Source: CAD feature listing. Evaluate the final solid. Frame: model axes, mm. A direction names the side the tool comes from. Give positions to 0.01 mm unless a question says otherwise; leave off trailing zeros. Write each loop counter-clockwise with the first axis right and the second up, starting at its lowest first coordinate (ties: lowest second). Pieces come first, ordered by that corner, then holes. Notation, with made-up numbers: (4.5, 30.5) -> (14.5, 30.5) arc R34 ccw to (14.5, 60.5) -> close; hole circle Ø2 at (19, 1.5). An arc over 180 degrees is marked (long way). Write item = value, one per line.
from build123d import *

# Parameters (mm, degrees)
BOSS_EXTRUDE1_DEPTH     = 7.3
CUT_EXTRUDE1_DEPTH      = 8
CUT_EXTRUDE2_DEPTH      = 8
CUT_EXTRUDE3_DEPTH      = 34.01953967
CUT_EXTRUDE3_DEPTH_BACK = 34.01953967
CHAMFER1_SIZE           = 0.7


with BuildPart() as part:
    # Sketch1 → Boss-Extrude1 (new body)
    with BuildSketch(Plane.XY):
        Polygon((0, 0), (19, 0), (19, 18), (10.45, 18), (10.45, 26), (8.55, 26), (8.55, 18), (0, 18), align=None)
    extrude(amount=BOSS_EXTRUDE1_DEPTH)

    # Sketch2 → Cut-Extrude1 (cut)
    with BuildSketch(Plane(origin=(0, 26, 0), x_dir=(1, 0, 0), z_dir=(0, 1, 0))):
        with BuildLine():
            Line((8.55, -0.95), (8.55, 0))
            Line((8.55, 0), (9.5, 0))
            ThreePointArc((9.5, 0), (8.828248558, -0.278248558), (8.55, -0.95))
        make_face()
    extrude(amount=-CUT_EXTRUDE1_DEPTH, mode=Mode.SUBTRACT)

    # Sketch3 → Cut-Extrude2 (cut)
    with BuildSketch(Plane(origin=(0, 26, 0), x_dir=(1, 0, 0), z_dir=(0, 1, 0))):
        with BuildLine():
            Line((9.5, 0), (10.45, 0))
            Line((10.45, 0), (10.45, -0.95))
            ThreePointArc((10.45, -0.95), (10.171751442, -0.278248558), (9.5, 0))
        make_face()
    extrude(amount=-CUT_EXTRUDE2_DEPTH, mode=Mode.SUBTRACT)

    # Sketch4 → Cut-Extrude3 (cut, two sides: drawn at the far end of the back side and taken through both)
    with BuildSketch(Plane(origin=(19, 0, 0), x_dir=(0, 0, -1), z_dir=(1, 0, 0)).offset(-CUT_EXTRUDE3_DEPTH_BACK)):
        with BuildLine():
            Line((-5.25, 14.8), (-5.25, 4))
            ThreePointArc((-5.25, 4), (-3.65, 2.4), (-2.05, 4))
            Line((-2.05, 4), (-2.05, 14.8))
            ThreePointArc((-2.05, 14.8), (-3.65, 16.4), (-5.25, 14.8))
        make_face()
    extrude(amount=CUT_EXTRUDE3_DEPTH + CUT_EXTRUDE3_DEPTH_BACK, mode=Mode.SUBTRACT)

    # Chamfer1
    chamfer1_edges = [part.edges().sort_by_distance(p)[0] for p in [
        (0, 18, 3.65),
        (8.55, 26, 4.125),
        (10.45, 26, 4.125),
        (19, 18, 3.65),
        (9.5, 26, 0),
    ]]
    chamfer(chamfer1_edges, length=CHAMFER1_SIZE)


solid = part.part
(1) Section query C-C (y = 12.25). Return loops of the section in (x, z), plus the area to 3 significant figures.
Values follow:
outline = (0, 0) -> (19, 0) -> (19, 2.05) -> (0, 2.05) -> close; (0, 5.25) -> (19, 5.25) -> (19, 7.3) -> (0, 7.3) -> close
area = 77.9 mm2
(2) Section query D-D (z = 6.25). Return loops of the section in (x, y).
Values follow:
outline = (0, 0) -> (19, 0) -> (19, 17.3) -> (18.3, 18) -> (10.45, 18) -> (10.45, 25.3) -> (9.75, 26) -> (9.25, 26) -> (8.55, 25.3) -> (8.55, 18) -> (0.7, 18) -> (0, 17.3) -> close
(3) Access query for faces 1 (the face through (8.55, 22, 4)), 2 (the face through (9.4, 16.4, 3.6)), 3 (the face through (10.45, 22, 4)), 4 (the face through (0, 9, 1)). Directions: +Z, -Z, +X, -X, +Y, -Y. A direction counts if a zero-diameter tool reaches every point of the face in a straight line with its end or side. Return the directions, or none.
Values follow:
face_1 = +Z, -Z, -X, +Y
face_2 = +X, -X
face_3 = +Z, -Z, +X, +Y
face_4 = +Z, -Z, -X, +Y, -Y
(4) First-contact query: pin 1 (4 mm diameter, centred on x = 15, z = 4, fed in from +Y); pin 2 (1.5 mm diameter, centred on y = 20.5, z = 4, fed in from -X); pin 3 (1.9 mm diameter, centred on y = 23, z = 3.5, fed in from -X). Flat tips, straight axial feed; report the tip coordinate or a pass-through.
Values follow:
pin_1 = 18
pin_2 = 8.55
pin_3 = 8.55
(5) Section query B-B (x = 11.5). Return loops of the section in (y, z), plus the area to 3 significant figures.
Values follow:
outline = (0, 0) -> (18, 0) -> (18, 7.3) -> (0, 7.3) -> close; hole (4, 2.05) -> (14.8, 2.05) arc R1.6 ccw to (14.8, 5.25) -> (4, 5.25) arc R1.6 ccw to start
area = 88.8 mm2
(6) Pull-direction query (Z, two-part tool) for faces 5 (the face through (9, 9, 5.25)), 6 (the face through (9, 10, 7.3)), 7 (the face through (4, 18, 4)); classes: pulls with the +Z half, pulls with the -Z half, needs draft (parallel to the pull), parting line crosses it, or undercut.
Values follow:
face_5 = undercut
face_6 = pulls with the +Z half
face_7 = needs draft
(7) Material intervals for line 1 (Z direction, x = 7, y = 11); line 2 (X direction, y = 22.5, z = 1.5), sorted ascending.
Values follow:
line_1 = 0 to 2.05, 5.25 to 7.3
line_2 = 8.55 to 10.45
(8) Section query A-A (z = 3.65). Return loops of the section in (x, y).
Values follow:
outline = (0, 0) -> (19, 0) -> (19, 2.4) -> (0, 2.4) -> close; (0, 16.4) -> (19, 16.4) -> (19, 17.3) -> (18.3, 18) -> (10.45, 18) -> (10.45, 25.3) -> (9.75, 26) -> (9.25, 26) -> (8.55, 25.3) -> (8.55, 18) -> (0.7, 18) -> (0, 17.3) -> close
